from build123d import *

# Parameters (mm, degrees)
SKETCH_2_W               = 8.3
SKETCH_2_H               = 4
EXTRUDE_1_DEPTH          = 8
SKETCH_3_W               = 10.1
SKETCH_3_H               = 4.8
EXTRUDE_2_DEPTH          = 0.4
CUT_EXTRUDE_1_DEPTH      = 14.350655415
CUT_EXTRUDE_1_DEPTH_BACK = 3
SKETCH_4_W               = 1
SKETCH_4_H               = 0.5
SKETCH_5_R               = 0.5
CUT_EXTRUDE_2_DEPTH      = 10


with BuildPart() as part:
    # 草图2 → 凸台-拉伸1 (new body)
    with BuildSketch(Plane.XY):
        with Locations((4.15, 2)):
            Rectangle(SKETCH_2_W, SKETCH_2_H)
    extrude(amount=EXTRUDE_1_DEPTH)

    # 草图3 → 凸台-拉伸2 (add)
    with BuildSketch(Plane.XY.offset(8)):
        with Locations((4.15, 2.4)):
            Rectangle(SKETCH_3_W, SKETCH_3_H)
    extrude(amount=EXTRUDE_2_DEPTH)

    # 草图4 → 切除-拉伸1 (cut, two sides: drawn at the far end of the back side and taken through both)
    with BuildSketch(Plane(origin=(0, 0, 0), x_dir=(-1, 0, 0), z_dir=(0, 0, -1)).offset(-CUT_EXTRUDE_1_DEPTH_BACK)):
        with Locations((-4.15, 3.75)):
            Rectangle(SKETCH_4_W, SKETCH_4_H)
        with Locations((-6.69, 3.75)):
            Rectangle(SKETCH_4_W, SKETCH_4_H)
        with Locations((-1.61, 3.75)):
            Rectangle(SKETCH_4_W, SKETCH_4_H)
    extrude(amount=CUT_EXTRUDE_1_DEPTH + CUT_EXTRUDE_1_DEPTH_BACK, mode=Mode.SUBTRACT)

    # 草图5 → 切除-拉伸2 (cut)
    with BuildSketch(Plane(origin=(0, 0, 0), x_dir=(-1, 0, 0), z_dir=(0, 0, -1))):
        with Locations((-6.684838564, 1)):
            Circle(SKETCH_5_R)
        with Locations((-4.144838564, 1)):
            Circle(SKETCH_5_R)
        with Locations((-1.615161436, 1)):
            Circle(SKETCH_5_R)
    extrude(amount=-CUT_EXTRUDE_2_DEPTH, mode=Mode.SUBTRACT)


solid = part.part
Geometry: final body of the model. Coordinates: model frame, mm. A direction names the side the tool comes from. Give positions to 0.01 mm unless a question says otherwise; leave off trailing zeros. Loops run counter-clockwise (first coordinate to the right, second up) from the corner with the lowest first, then second, coordinate; pieces in that order, holes last. Notation, with made-up numbers: (-30.5, 65.5) - (-12.5, 65.5) arc R28 ccw to (-12.5, 84.5) - close; hole circle Ø2 at (24.5, 77.5). An arc over 180 degrees is marked (long way). Answer as CSV lines item,"result". Start each with the question number.
1. Section A-A, the plane y = 1. Return loops of the section in (x, z).
2. Section D-D, the plane x = 5.5. Return loops of the section in (y, z).
3. Ray query, L1, parallel to X at y = 1.15, z = 8.25; L2, parallel to X at y = 1.2, z = 2.75; L3, parallel to Y at x = 5.5, z = 0.5. Return the intervals inside material, ascending.
4. Draft query along Y for faces 5 (the face through (0, 2, 4)), 6 (the face through (1.72, 0.51, 4.14)), 7 (the face through (4, 3.5, 2)). Return one class per face: released by +Y, released by -Y, zero draft, split by the parting line, or undercut.
5. Section C-C, the plane y = 3.85. Return loops of the section in (x, z).
6. Reachability of faces 1 (the face through (8.3, 2, 4)), 2 (the face through (4, 4, 4)), 3 (the face through (7, 3.5, 2)), 4 (the face through (4.644, 1.022, 4.141)) from +Z, -Z, +X, -X, +Y, -Y: full face, straight path, thin tool, end or side. Return the list, or none.
7. Pin query (flat end, axial travel): P1, Ø0.6, axis at y = 4, z = 1, coming from the -X side; P2, Ø0.6, axis at y = 4, z = 1, coming from the +X side; P3, Ø0.5, axis at x = 4, z = 1, coming from the +Y side. Return the tip coordinate at first contact, or that it passes through.
8. Section B-B, the plane z = 0.5. Return loops of the section in (x, y).
Answers:
1,outline,"(-0.9, 8) - (0, 8) - (0, 0) - (1.12, 0) - (1.12, 8.4) - (-0.9, 8.4) - close; (2.12, 0) - (3.64, 0) - (3.64, 8.4) - (2.12, 8.4) - close; (4.64, 0) - (6.18, 0) - (6.18, 8.4) - (4.64, 8.4) - close; (7.18, 0) - (8.3, 0) - (8.3, 8) - (9.2, 8) - (9.2, 8.4) - (7.18, 8.4) - close"
2,outline,"(0, 0) - (4, 0) - (4, 8) - (4.8, 8) - (4.8, 8.4) - (0, 8.4) - close"
3,L1,"x = -0.9 to 1.14, 2.09 to 3.67, 4.62 to 6.21, 7.16 to 9.2"
3,L2,"x = 0 to 1.16, 2.07 to 3.69, 4.6 to 6.23, 7.14 to 8.3"
3,L3,"y = 0 to 4"
4,face 5,"zero draft"
4,face 6,"undercut"
4,face 7,"released by +Y"
5,outline,"(-0.9, 8) - (0, 8) - (0, 0) - (1.11, 0) - (1.11, 3) - (2.11, 3) - (2.11, 0) - (3.65, 0) - (3.65, 3) - (4.65, 3) - (4.65, 0) - (6.19, 0) - (6.19, 3) - (7.19, 3) - (7.19, 0) - (8.3, 0) - (8.3, 8) - (9.2, 8) - (9.2, 8.4) - (-0.9, 8.4) - close"
6,face 1,"-Z, +X, +Y, -Y"
6,face 2,"-Z, +X, -X, +Y"
6,face 3,"-Z, +Y"
6,face 4,"+Z, -Z"
7,P1,"stops at x = 0"
7,P2,"stops at x = 8.3"
7,P3,"stops at y = 3.5"
8,outline,"(0, 0) - (8.3, 0) - (8.3, 4) - (7.19, 4) - (7.19, 3.5) - (6.19, 3.5) - (6.19, 4) - (4.65, 4) - (4.65, 3.5) - (3.65, 3.5) - (3.65, 4) - (2.11, 4) - (2.11, 3.5) - (1.11, 3.5) - (1.11, 4) - (0, 4) - close; hole circle Ø1 at (1.62, 1); hole circle Ø1 at (4.14, 1); hole circle Ø1 at (6.68, 1)"
